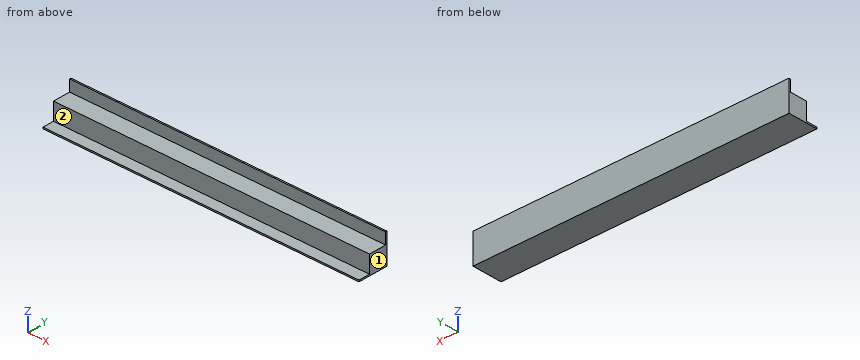
from build123d import *

# Parameters (mm, degrees)
SKETCH2_W           = 420
SKETCH2_H           = 40
BOSS_EXTRUDE1_DEPTH = 40
SKETCH3_W           = 38
SKETCH3_H           = 38
CUT_EXTRUDE1_DEPTH  = 1000
SKETCH4_W           = 23
SKETCH4_H           = 23
BOSS_EXTRUDE2_DEPTH = 420


with BuildPart() as part:
    # Sketch2 → Boss-Extrude1 (new body)
    with BuildSketch(Plane.XY):
        with Locations((-6.593186373, 82.705410822)):
            Rectangle(SKETCH2_W, SKETCH2_H)
    extrude(amount=BOSS_EXTRUDE1_DEPTH)

    # Sketch3 → Cut-Extrude1 (cut)
    with BuildSketch(Plane.ZY.offset(216.593186373)):
        with Locations((21, 81.705410822)):
            Rectangle(SKETCH3_W, SKETCH3_H)
    extrude(amount=-CUT_EXTRUDE1_DEPTH, mode=Mode.SUBTRACT)

    # Sketch4 → Boss-Extrude2 (add)
    with BuildSketch(Plane.ZY.offset(216.593186373)):
        with Locations((13.5, 89.205410822)):
            Rectangle(SKETCH4_W, SKETCH4_H)
    extrude(amount=-BOSS_EXTRUDE2_DEPTH)


solid = part.part
CAD build for the part. Positions are in the model's coordinates, mm. Face numbers are marked on the shaded views. A direction names the side the tool comes from. Coordinates: 2 decimals unless noted, no trailing zeros. Loops run counter-clockwise (first coordinate to the right, second up) from the corner with the lowest first, then second, coordinate; pieces in that order, holes last. Notation, with made-up numbers: (-34.75, 3.5) - (-30.75, 3.5) arc R20 ccw to (-30.75, 35.5) - close; hole circle Ø11 at (-3.75, -8). An arc over 180 degrees is marked (long way). Use one line per item in the form item = value. Start each with the question number.
1) Band-saw the part on A-A (x = -33). Give the cut face in (y, z), and give its area (3 significant figures).
2) Drill centre lines: L1, parallel to Y at x = -103.5, z = 35; L2, parallel to Z at x = 51, y = 68; L3, parallel to Z at x = 23, y = 83.5. Where is each one in solid material? Low to high. Write a range as from..to.
3) Tool access for the marked faces 1 and 2: list every direction of +Z, -Z, +X, -X, +Y, -Y with a clear straight run to the whole face (end or side of a thin tool).
4) Flat gauge pins, fed straight in: pin 1 (3 mm diameter, centred on x = -44, z = 34.5, fed in from -Y); pin 2 (11.5 mm diameter, centred on x = -91.5, z = 11.5, fed in from -Y); pin 3 (12 mm diameter, centred on x = 57.5, y = 68.5, fed in from +Z). Where does each tip first touch, or does it go through?
5) Band-saw the part on C-C (y = 83.5). Give the cut face in (x, z).
6) Band-saw the part on B-B (z = 18.5). Give the cut face in (x, y), and give its area (3 significant figures).
Check values:
q1.outline = (62.71, 0) - (102.71, 0) - (102.71, 40) - (100.71, 40) - (100.71, 25) - (77.71, 25) - (77.71, 2) - (62.71, 2) - close
q1.area = 685 mm2
q2.L1 = 100.71..102.71
q2.L2 = 0..2
q2.L3 = 0..25
q3.face_1 = +Z, -Z, +X, +Y, -Y
q3.face_2 = +Z, +X, -X, -Y
q4.pin_1 = 100.71
q4.pin_2 = 77.71
q4.pin_3 = 2
q5.outline = (-216.59, 0) - (203.41, 0) - (203.41, 25) - (-216.59, 25) - close
q6.outline = (-216.59, 77.71) - (203.41, 77.71) - (203.41, 102.71) - (-216.59, 102.71) - close
q6.area = 10,500 mm2
